Here's how the part is built. I have some questions about the finished solid (model axes, mm). Face numbers are marked on the shaded views. Round coordinates to 2 decimals unless told otherwise and drop trailing zeros. Loops run counter-clockwise (first coordinate to the right, second up) from the corner with the lowest first, then second, coordinate; pieces in that order, holes last. Notation, with made-up numbers: (18, -22) - (28, -22) arc R18 ccw to (28, -13) - close; hole circle Ø7 at (-31.75, 24). An arc over 180 degrees is marked (long way). Answer as a JSON object with one key per item and string values. Group by question number.
1) Will this pin go through, and if not, where does the flat tip stop? P1, Ø5, axis at x = 32.5, z = 4, coming from the -Y side.
2) I want a section at A-A, the plane z = -20. Please give me the cut outline in (x, y) (3 decimals).
3) I want a section at D-D, the plane y = 10.5. Please give me the cut outline in (x, z), then the cut area to 3 significant figures.
4) If I drill on line 1 along Z through (x, y) = (0, 43); line 2 along Y through (x, z) = (-53, 3); line 3 along Y through (x, z) = (-42, -24.5), over which ranges is the centre line in solid material (lowest first)? Write a range as [from, to].
5) I want a section at B-B, the plane x = 0. Please give me the cut outline in (y, z), then the cut area to 3 significant figures.
6) If we mould it in two halves opening along Y, with no side actions, what happens to the marked faces 1, 2 and 3? For each: pulls with the +Y half, pulls with the -Y half, needs draft (parallel to the pull), parting line crosses it, or undercut.
7) I want a section at C-C, the plane y = 27.5. Please give me the cut outline in (x, z), then the cut area to 3 significant figures.
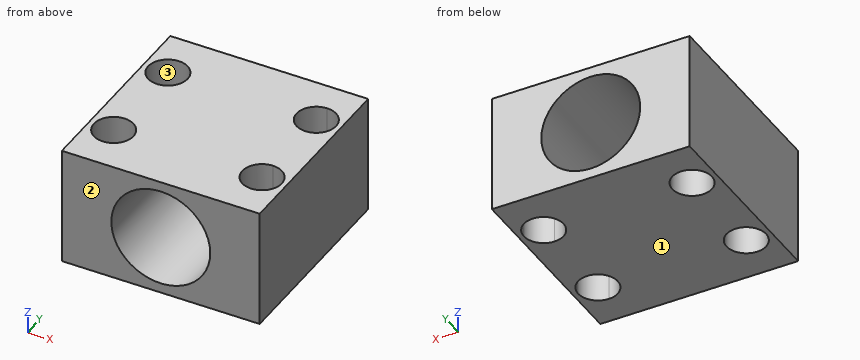
from build123d import *

# Parameters (mm, degrees)
SKETCH2_W           = 127
SKETCH2_H           = 76.2
SKETCH2_R           = 31.75
BOSS_EXTRUDE1_DEPTH = 127
SKETCH3_R           = 12.7
CUT_EXTRUDE1_DEPTH  = 127


with BuildPart() as part:
    # Sketch2 → Boss-Extrude1 (new body)
    with BuildSketch(Plane(origin=(0, 0, 0), x_dir=(1, 0, 0), z_dir=(0, 1, 0))):
        Rectangle(SKETCH2_W, SKETCH2_H)
        Circle(SKETCH2_R, mode=Mode.SUBTRACT)
    extrude(amount=BOSS_EXTRUDE1_DEPTH)

    # Sketch3 → Cut-Extrude1 (cut)
    with BuildSketch(Plane.XY.offset(38.1)):
        with BuildLine():
            ThreePointArc((60.325, 95.25), (56.605256121, 104.230256121), (47.625, 107.95))
            Line((47.625, 107.95), (47.625, 82.55))
            ThreePointArc((47.625, 82.55), (56.605256121, 86.269743879), (60.325, 95.25))
        make_face()
        with BuildLine():
            Line((47.625, 82.55), (47.625, 107.95))
            ThreePointArc((47.625, 107.95), (34.925, 95.25), (47.625, 82.55))
        make_face()
        with BuildLine():
            ThreePointArc((60.325, 31.75), (56.605256121, 40.730256121), (47.625, 44.45))
            Line((47.625, 44.45), (47.625, 19.05))
            ThreePointArc((47.625, 19.05), (56.605256121, 22.769743879), (60.325, 31.75))
        make_face()
        with BuildLine():
            Line((47.625, 19.05), (47.625, 44.45))
            ThreePointArc((47.625, 44.45), (34.925, 31.75), (47.625, 19.05))
        make_face()
        with Locations((-47.625, 31.75)):
            Circle(SKETCH3_R)
        with Locations((-47.625, 95.25)):
            Circle(SKETCH3_R)
    extrude(amount=-CUT_EXTRUDE1_DEPTH, mode=Mode.SUBTRACT)


solid = part.part
Outcome:
{
 "1": {"P1": "y = 0"},
 "2": {"outline": "(-63.5, 0) - (-24.659, 0) - (-24.659, 127) - (-63.5, 127) - close; (24.659, 0) - (63.5, 0) - (63.5, 127) - (24.659, 127) - close; hole circle Ø25.4 at (-47.625, 31.75); hole circle Ø25.4 at (-47.625, 95.25); hole circle Ø25.4 at (47.625, 31.75); hole circle Ø25.4 at (47.625, 95.25)"},
 "3": {"outline": "(-63.5, -38.1) - (63.5, -38.1) - (63.5, 38.1) - (-63.5, 38.1) - close; hole circle Ø63.5 at (0, 0)", "area": "6,510 mm^2"},
 "4": {"line 1": "[-38.1, -31.75], [31.75, 38.1]", "line 2": "[0, 20.24], [43.26, 83.74], [106.76, 127]", "line 3": "[0, 20.36], [43.14, 83.86], [106.64, 127]"},
 "5": {"outline": "(0, -38.1) - (127, -38.1) - (127, -31.75) - (0, -31.75) - close; (0, 31.75) - (127, 31.75) - (127, 38.1) - (0, 38.1) - close", "area": "1,610 mm^2"},
 "6": {"face 1": "needs draft", "face 2": "pulls with the -Y half", "face 3": "undercut"},
 "7": {"outline": "(-63.5, -38.1) - (-59.59, -38.1) - (-59.59, 38.1) - (-63.5, 38.1) - close; (-35.66, -38.1) - (35.66, -38.1) - (35.66, 38.1) - (-35.66, 38.1) - close; (59.59, -38.1) - (63.5, -38.1) - (63.5, 38.1) - (59.59, 38.1) - close; hole circle Ø63.5 at (0, 0)", "area": "2,860 mm^2"}
}
